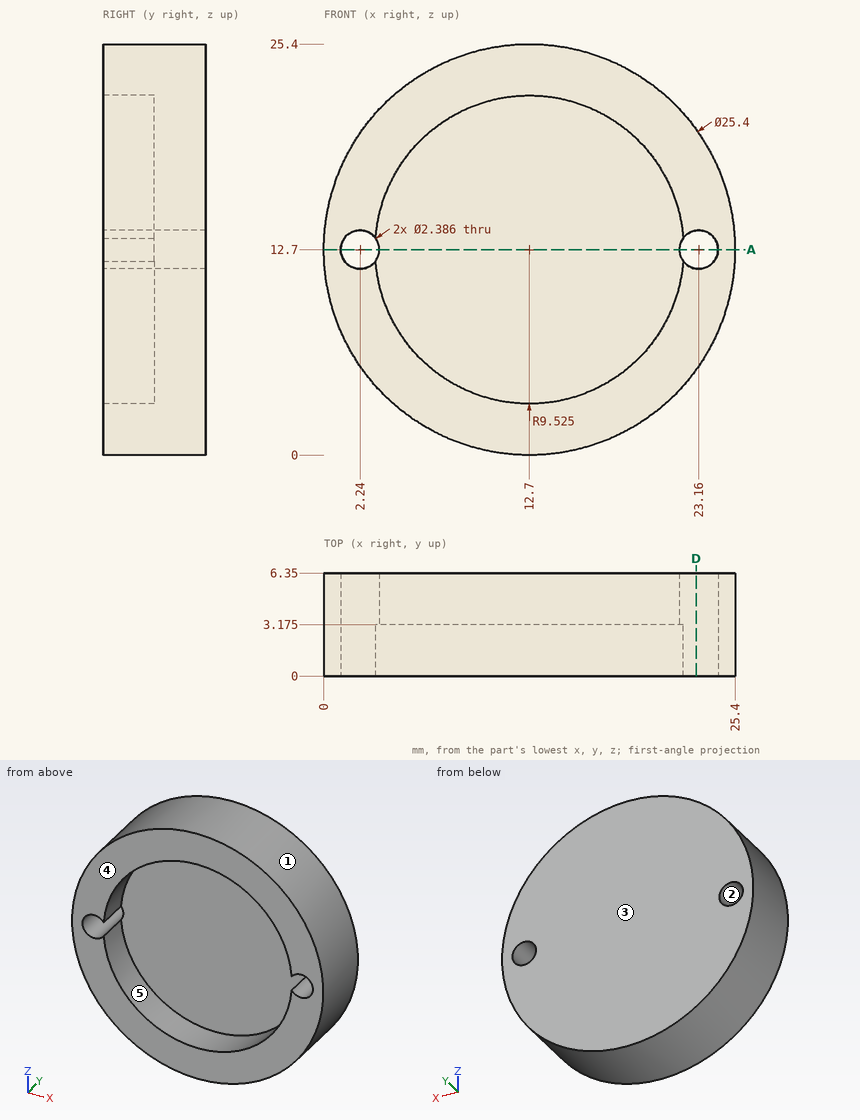
Answer from the drawing. Dimensions are ordinates in mm from the lowest x, y and z of the part. A direction names the side the tool comes from. Coordinates: 2 decimals unless noted, no trailing zeros. Loops run counter-clockwise (first coordinate to the right, second up) from the corner with the lowest first, then second, coordinate; pieces in that order, holes last. Notation, with made-up numbers: (10, 18) - (24, 18) arc R29 cw to (24, 47) - close; hole circle Ø11 at (2.25, -12). An arc over 180 degrees is marked (long way). Use a Markdown table: item, result.
Item 1: Given pin 1 Ø2 at (x, y) = (10.5, 1) entering from -Z; pin 2 Ø1 at (x, y) = (5, 5) entering from -Z; pin 3 Ø5.5 at (x, z) = (13.5, 9.5) entering from -Y (3 decimals), each flat-ended and moving along its own axis, determine where each tip first touches the part or whether it passes through.
Evaluation:
| item | result |
|---|---|
| pin 1 | stops at z = 0.06 |
| pin 2 | stops at z = 2.24 |
| pin 3 | stops at y = 3.175 |
Item 2: The mould has two halves that part along Z. Classify the marked faces 1, 2 and 3: +Z half, -Z half, draft (parallel to the pull), parting line (faces both ways), or undercut.
Evaluation:
| item | result |
|---|---|
| face 1 | parting line |
| face 2 | undercut |
| face 3 | draft |
Item 3: Find section A-A, the plane z = 12.7. State how many separate pieces and enclosed holes the cut face has.
Evaluation:
| item | result |
|---|---|
| separate pieces | 3 |
| enclosed holes | 0 |
Item 4: Find section D-D, the plane x = 23. Determine the outline of the cut face in (y, z).
Evaluation:
| item | result |
|---|---|
| outline | (0, 5.27) - (6.35, 5.27) - (6.35, 11.52) - (0, 11.52) - close; (0, 13.88) - (6.35, 13.88) - (6.35, 20.13) - (0, 20.13) - close |
Item 5: For the marked faces 4 and 5, determine the directions among +Z, -Z, +X, -X, +Y, -Y from which every point of the face is accessible in a straight line to the end or side of a thin tool.
Evaluation:
| item | result |
|---|---|
| face 4 | +Z, -Z, +X, -X, -Y |
| face 5 | -Y |
Item 6: Consider probe 1 along X at (y, z) = (2.25, 12.7); probe 2 along Z at (x, y) = (23.5, 3) (1 decimal); probe 3 along Z at (x, y) = (23, 5) (1 decimal). Determine where each line is inside the solid, lowest interval first. Write a range as from..to.
Evaluation:
| item | result |
|---|---|
| probe 1 | x = 0..1.05, 24.35..25.4 |
| probe 2 | z = 6..11.6, 13.8..19.4 |
| probe 3 | z = 5.3..11.5, 13.9..20.1 |
